The model under review builds one solid part; all positions refer to its coordinate system, in mm. A direction names the side the tool comes from. Round coordinates to 2 decimals unless told otherwise and drop trailing zeros. Order: outer loops, then holes, each group sorted by start corner. A loop starts at its lowest first (then second) coordinate and runs counter-clockwise, first axis right, second up. Notation, with made-up numbers: M 61,50 L 95,50 A17 cw 95,74 Z; hole C 24,-22.5 d4. An arc over 180 degrees is marked long. Answer as a JSON object with one key per item and string values. Group by question number.
1. Add section B-B on y = 79.5. State the section outline as (x, z) points.
2. Mouldability with a two-part tool opening along X and no side actions: class faces 1 (the face through (-15.61, 62.01, 22.97)), 2 (the face through (0, 98, 32)), 3 (the face through (8.43, 53.35, 22.97)) as released by +X, released by -X, zero draft, split by the parting line, or undercut.
3. Add section C-C on z = 24. State the section outline as (x, y) points, and give its area (3 significant figures).
4. To check wall thickness, follow probe 1 along Z at (x, y) = (-5, 87); probe 2 along X at (y, z) = (61, 1); probe 3 along Y at (x, z) = (0, 58). State the ranges of each line that lie inside material, in increasing order. Write a range as [from, to].
5. Add section D-D on z = 50.5. State the section outline as (x, y) points.
6. Add section A-A on x = 0. State the section outline as (y, z) points.
7. Clearance check with flat-ended pins moving along their axes: P1, Ø1, axis at x = -5.5, z = 14, coming from the -Y side; P2, Ø12, axis at x = 1.5, y = 79, coming from the +Z side; P3, Ø3, axis at x = -8.5, z = 22, coming from the -Y side. State where each tip first meets the part, or that it passes through.
8. Machinability: for faces 4 (the face through (-4, 71, 25)), 5 (the face through (0, 94, 12)), 6 (the face through (0, 96, 62.27)), which of the approach directions +Z, -Z, +X, -X, +Y, -Y give a long, thin tool a straight path to every point of the face, cutting with its end or side? Answer none if there is none.
```python
from build123d import *

# Parameters (mm, degrees)
PAD009_DEPTH         = 20
SKETCH017_R          = 3
POCKET005_DEPTH      = 62.271
SKETCH018_R          = 1.5
POCKET006_DEPTH      = 0.001
POCKET006_DEPTH_BACK = 62.271


with BuildPart() as part:
    # Sketch016 → Pad009 (new body, symmetric)
    with BuildSketch(Plane.YZ):
        Polygon((0, 62.27), (0, 0), (-49, 0), (-49, 4), (-4, 4), (-4, 21), (-49, 21), (-49, 25), (-4, 25), (-4, 62.27), align=None)
    extrude(amount=PAD009_DEPTH, both=True)

    # Sketch017 → Pocket005 (cut, through all)
    with BuildSketch(Plane.XY):
        with Locations((0, -37)):
            Circle(SKETCH017_R)
    extrude(amount=POCKET005_DEPTH, mode=Mode.SUBTRACT)

    # Sketch018 → Pocket006 (cut, two sides)
    with BuildSketch(Plane.XY) as pocket006_sk:
        with Locations((-14.5, -37)):
            Circle(SKETCH018_R)
        with BuildLine():
            ThreePointArc((-20, -37), (-13.535443, -45.691314), (-3.221276, -49))
            Line((-3.221276, -49), (-2.229993, -49))
            ThreePointArc((-2.229993, -49), (8.544467, -44.53401), (13, -33.755222))
            Line((13, -33.755222), (12.980003, -13.146812))
            ThreePointArc((20, -6.12), (15.033703, -8.178519), (12.980003, -13.146812))
            Line((20, -6.12), (20, -54.21))
            Line((20, -54.21), (-20, -54.21))
            Line((-20, -37), (-20, -54.21))
        make_face()
    extrude(amount=-POCKET006_DEPTH, mode=Mode.SUBTRACT)
    extrude(pocket006_sk.sketch, amount=POCKET006_DEPTH_BACK, mode=Mode.SUBTRACT)


with BuildPart() as part_1:
    # Body004 placement: moved
    add(part.part.moved(Location((0, 98, 0))))


solid = part_1.part
```
Recorded:
{
 "1": {"outline": "M -20,0 L 12.99,0 L 12.99,4 L -20,4 Z; M -20,21 L 12.99,21 L 12.99,25 L -20,25 Z"},
 "2": {"face 1": "undercut", "face 2": "zero draft", "face 3": "released by +X"},
 "3": {"outline": "M -20,61 A17.73 ccw -3.22,49 L -2.23,49 A15.23 ccw 13,64.24 L 12.98,84.85 A7.02 cw 20,91.88 L 20,98 L -20,98 Z; hole C -14.5,61 d3; hole C 0,61 d6", "area": "1,530 mm²"},
 "4": {"probe 1": "z = [0, 4], [21, 25]", "probe 2": "x = [-20, -16], [-13, -3], [3, 12.65]", "probe 3": "y = [94, 98]"},
 "5": {"outline": "M -20,94 L 20,94 L 20,98 L -20,98 Z"},
 "6": {"outline": "M 49.16,0 L 58,0 L 58,4 L 49.16,4 Z; M 49.16,21 L 58,21 L 58,25 L 49.16,25 Z; M 64,0 L 98,0 L 98,62.27 L 94,62.27 L 94,25 L 64,25 L 64,21 L 94,21 L 94,4 L 64,4 Z"},
 "7": {"P1": "stops at y = 94", "P2": "stops at z = 25", "P3": "stops at y = 49.41"},
 "8": {"face 4": "+Z, +X, -X, -Y", "face 5": "+X, -X, -Y", "face 6": "+Z, +X, -X, +Y, -Y"}
}
